Design review of the part built by this model. Coordinates are the model's own, in mm. A direction names the side the tool comes from. Round coordinates to 2 decimals unless told otherwise and drop trailing zeros. Order: outer loops, then holes, each group sorted by start corner. A loop starts at its lowest first (then second) coordinate and runs counter-clockwise, first axis right, second up. Notation, with made-up numbers: (-10, 8.5) - (34, 8.5) arc R25 cw to (34, 41.5) - close; hole circle Ø11 at (-1.75, 56.5). An arc over 180 degrees is marked (long way). Use CSV: the item, a comma, the result in double quotes.
from build123d import *

# Parameters (mm, degrees)
F0_W      = 14
F0_H      = 44
F1_DEPTH  = 18
F2_W      = 14
F2_H      = 10
F3_DEPTH  = 16
F4_R      = 1.625
F5_DEPTH  = 2
F6_R      = 2.5
F7_DEPTH  = 34
F6_R_2    = 4.5
F8_DEPTH  = 31.5
F6_R_3    = 5
F9_DEPTH  = 19.5
F11_DEPTH = 34
F12_R     = 1.5


with BuildPart() as f1:
    # F0 (on Top) → F1 (new body)
    with BuildSketch(Plane.XY):
        with Locations((7, 22)):
            Rectangle(F0_W, F0_H)
    extrude(amount=F1_DEPTH)

    # F2 (on face) → F3 (cut)
    with BuildSketch(Plane.XY.offset(18)):
        with Locations((7, 39)):
            Rectangle(F2_W, F2_H)
    extrude(amount=-F3_DEPTH, mode=Mode.SUBTRACT)

    # F4 (on face) → F5 (cut, through all)
    with BuildSketch(Plane.XY.offset(2)):
        with Locations((7, 39.625)):
            Circle(F4_R)
    extrude(amount=-F5_DEPTH, mode=Mode.SUBTRACT)

    # F6 (on face) → F7 (cut, through all)
    with BuildSketch(Plane(origin=(0, 34, 0), x_dir=(-1, 0, 0), z_dir=(0, 1, 0))):
        with Locations((-7, 12.5)):
            Circle(F6_R)
    extrude(amount=-F7_DEPTH, mode=Mode.SUBTRACT)

    # F6 (on face) → F8 (cut)
    with BuildSketch(Plane(origin=(0, 34, 0), x_dir=(-1, 0, 0), z_dir=(0, 1, 0))):
        with Locations((-7, 12.5)):
            Circle(F6_R_2)
        with Locations((-7, 12.5)):
            Circle(F6_R, mode=Mode.SUBTRACT)
    extrude(amount=-F8_DEPTH, mode=Mode.SUBTRACT)

    # F6 (on face) → F9 (cut)
    with BuildSketch(Plane(origin=(0, 34, 0), x_dir=(-1, 0, 0), z_dir=(0, 1, 0))):
        with Locations((-7, 12.5)):
            Circle(F6_R_3)
        with Locations((-7, 12.5)):
            Circle(F6_R_2, mode=Mode.SUBTRACT)
    extrude(amount=-F9_DEPTH, mode=Mode.SUBTRACT)

    # F10 (on face) → F11 (cut, through all)
    with BuildSketch(Plane(origin=(0, 34, 0), x_dir=(-1, 0, 0), z_dir=(0, 1, 0))):
        with BuildLine():
            ThreePointArc((-4.5, 16.8301270189), (-7, 17.5), (-9.5, 16.8301270189))
            Line((-9.5, 16.8301270189), (-9.5, 12.5))
            ThreePointArc((-9.5, 12.5), (-7, 15), (-4.5, 12.5))
            Line((-4.5, 12.5), (-4.5, 16.8301270189))
        make_face()
        with BuildLine():
            Line((-4.5, 18), (-9.5, 18))
            Line((-9.5, 18), (-9.5, 16.8301270189))
            ThreePointArc((-9.5, 16.8301270189), (-7, 17.5), (-4.5, 16.8301270189))
            Line((-4.5, 16.8301270189), (-4.5, 18))
        make_face()
    extrude(amount=-F11_DEPTH, mode=Mode.SUBTRACT)

    # F12
    f12_edges = [f1.edges().sort_by_distance(p)[0] for p in [
        (0, 44, 1),
        (14, 44, 1),
        (4.5, 17, 18),
        (9.5, 17, 18),
        (14, 0, 9),
        (0, 0, 9),
        (0, 34, 10),
        (14, 34, 10),
    ]]
    fillet(f12_edges, radius=F12_R)


solid = f1.part
1) We need section A-A (z = 11.5). Give the boundary of the cut face in (x, y).
Data:
outline,"(0, 1.5) arc R1.5 ccw to (1.5, 0) - (4.71, 0) - (4.71, 2.5) - (2.61, 2.5) - (2.61, 14.5) - (2.1, 14.5) - (2.1, 34) - (1.5, 34) arc R1.5 ccw to (0, 32.5) - close; (9.29, 0) - (12.5, 0) arc R1.5 ccw to (14, 1.5) - (14, 32.5) arc R1.5 ccw to (12.5, 34) - (11.9, 34) - (11.9, 14.5) - (11.39, 14.5) - (11.39, 2.5) - (9.29, 2.5) - close"
2) We need section B-B (x = 7). Give the boundary of the cut face in (y, z), then the cut area to 3 significant figures.
Data:
outline,"(0, 0) - (38, 0) - (38, 2) - (34, 2) - (34, 7.5) - (14.5, 7.5) - (14.5, 8) - (2.5, 8) - (2.5, 10) - (0, 10) - close; (41.25, 0) - (44, 0) - (44, 2) - (41.25, 2) - close"
area,"281 mm2"
3) We need section C-C (y = 30). Give the boundary of the cut face in (x, z).
Data:
outline,"(0, 0) - (14, 0) - (14, 18) - (11, 18) arc R1.5 ccw to (9.53, 16.81) arc R5 cw (long way) to (4.47, 16.81) arc R1.5 ccw to (3, 18) - (0, 18) - close"
4) To check wall thickness, follow L1, parallel to Y at x = 7, z = 1; L2, parallel to X at y = 26.5, z = 12.75; L3, parallel to X at y = 10.75, z = 12.5. State the ranges of each line that lie inside material, in increasing order. Write a range as from..to.
Data:
L1,"y = 0..38, 41.25..44"
L2,"x = 0..2.01, 11.99..14"
L3,"x = 0..2.5, 11.5..14"
5) The part is to be moulded in two halves that separate along X. For faces 1 (the face through (9.93, 16.76, 17.55)), 2 (the face through (12, 17, 18)), 3 (the face through (13.57, 43.55, 1.01)), say which applies: +X half, -X half, draft (parallel to the pull), parting line (faces both ways), or undercut.
Data:
face 1,"undercut"
face 2,"draft"
face 3,"+X half"
6) We need section D-D (z = 9.5). Give the boundary of the cut face in (x, y).
Data:
outline,"(0, 1.5) arc R1.5 ccw to (1.5, 0) - (12.5, 0) arc R1.5 ccw to (14, 1.5) - (14, 32.5) arc R1.5 ccw to (12.5, 34) - (11, 34) - (11, 14.5) - (10.35, 14.5) - (10.35, 2.5) - (3.65, 2.5) - (3.65, 14.5) - (3, 14.5) - (3, 34) - (1.5, 34) arc R1.5 ccw to (0, 32.5) - close"
7) Insertion check: pin 1 Ø3.5 at (x, y) = (10.5, 37) entering from +Z; pin 2 Ø5.5 at (x, z) = (6.5, 8) entering from +Y; pin 3 Ø6 at (x, z) = (7.5, 11.5) entering from +Y. Each pin has a flat end and moves straight along its axis. Give the tip position at first contact, or say it passes through.
Data:
pin 1,"stops at z = 2"
pin 2,"stops at y = 34"
pin 3,"stops at y = 2.5"
8) For faces 4 (the face through (13.57, 33.55, 9.89)), 5 (the face through (4.5, 2, 15)), 6 (the face through (7, 34, 7)), 7 (the face through (7, 9, 8)), 8 (the face through (0.43, 33.55, 9.89)), list the 3-axis set-ups (+Z, -Z, +X, -X, +Y, -Y) from which the entire face can be reached by the end or side of a thin tool; tool diameter is ignored.
Data:
face 4,"+Z, +X, +Y"
face 5,"+Z, +Y, -Y"
face 6,"+Z, +X, -X, +Y"
face 7,"+Y"
face 8,"+Z, -X, +Y"
